Could you check a few things on this model? Use its own coordinates, in mm. Give positions to 0.01 mm unless a question says otherwise; leave off trailing zeros. Use a Markdown table: item, result. Add a question column.
Item 1: If I drill on L1, parallel to X at y = 0.85, z = 8.89; L2, parallel to X at y = 0.15, z = 8.5; L3, parallel to X at y = 0.25, z = -10.5, over which ranges is the centre line in solid material (lowest first)? Write a range as from..to.
Item 2: I'm going to push a flat-ended pin straight in: pin 1 Ø0.8 at (x, z) = (23.37, 2.43) entering from -Y. Where does the tip first touch, or does it pass through?
Item 3: Suppose I cut it at A-A on y = 0.9. Count the separate pieces of the cut face and the enclosed holes in it, plus the area to 3 significant figures.
Item 4: If we mould it in two halves opening along Z, with no side actions, what happens to faces 1 (the face through (-20.32, 0.77, -2.68)), 2 (the face through (0, 1, 11.43)), 3 (the face through (25.4, 1, 0))? For each: released by +Z, released by -Z, zero draft, split by the parting line, or undercut.
from build123d import *

# Parameters (mm, degrees)
SKETCH1_W                 = 50.8
SKETCH1_H                 = 22.86
BOSS_EXTRUDE1_DEPTH       = 1.57
F_1_16_0_1_DOWEL_HOLE1_D  = 2.54
FILLET1_R                 = 2.54
F_1_16_0_04_DOWEL_HOLE3_D = 1.016
LPATTERN6_COUNT           = 4
LPATTERN6_PITCH           = 2.54
LPATTERN6_COUNT_DIR2      = 2
LPATTERN6_PITCH_DIR2      = 2.54
LPATTERN7_COUNT           = 2
LPATTERN7_PITCH           = 2.54
LPATTERN7_COUNT_DIR2      = 4
LPATTERN7_PITCH_DIR2      = 2.54
LPATTERN8_COUNT           = 2
LPATTERN8_PITCH           = 41.656
LPATTERN8_COPY_1_D        = 1.016
LPATTERN8_COPY_2_D        = 1.016
LPATTERN8_COPY_3_D        = 1.016
LPATTERN8_COPY_4_D        = 1.016
LPATTERN8_COPY_5_D        = 1.016
LPATTERN8_COPY_6_D        = 1.016
LPATTERN8_COPY_7_D        = 1.016
LPATTERN8_COPY_8_D        = 1.016
LPATTERN8_COPY_9_D        = 1.016
LPATTERN8_COPY_10_D       = 1.016
LPATTERN8_COPY_11_D       = 1.016
LPATTERN8_COPY_12_D       = 1.016
LPATTERN8_COPY_13_D       = 1.016
LPATTERN8_COPY_14_D       = 1.016


with BuildPart() as part:
    # Sketch1 → Boss-Extrude1 (new body)
    with BuildSketch(Plane(origin=(0, 0, 0), x_dir=(1, 0, 0), z_dir=(0, 1, 0))):
        Rectangle(SKETCH1_W, SKETCH1_H)
    extrude(amount=BOSS_EXTRUDE1_DEPTH)

    # 1/16 (0.1) Dowel Hole1 (through all)
    with Locations(Plane(origin=(0, 1.57, 0), x_dir=(1, 0, 0), z_dir=(0, 1, 0))):
        with Locations((-22.86, 8.89), (22.86, 8.89), (22.86, -8.89), (-22.86, -8.89)):
            Hole(F_1_16_0_1_DOWEL_HOLE1_D / 2)

    # Fillet1
    fillet1_edges = [part.edges().sort_by_distance(p)[0] for p in [
        (25.4, 0.785, 11.43),
        (-25.4, 0.785, 11.43),
        (-25.4, 0.785, -11.43),
        (25.4, 0.785, -11.43),
    ]]
    fillet(fillet1_edges, radius=FILLET1_R)

    # 1/16 (0.04) Dowel Hole3 (through all)
    with Locations(Plane(origin=(0, 1.57, 0), x_dir=(1, 0, 0), z_dir=(0, 1, 0))):
        with Locations((-20.828, -4.965370827)):
            f_1_16_0_04_dowel_hole3 = Hole(F_1_16_0_04_DOWEL_HOLE3_D / 2)

    # LPattern6: 1_16 _0.04_ Dowel Hole3 4 × 2
    with Locations(*[(-j * LPATTERN6_PITCH_DIR2, 0, -i * LPATTERN6_PITCH) for i in range(LPATTERN6_COUNT) for j in range(LPATTERN6_COUNT_DIR2) if (i, j) != (0, 0)]):
        add(f_1_16_0_04_dowel_hole3, mode=Mode.SUBTRACT)

    # LPattern7: 1_16 _0.04_ Dowel Hole3 2 × 4
    with Locations(*[(i * LPATTERN7_PITCH, 0, -j * LPATTERN7_PITCH_DIR2) for i in range(LPATTERN7_COUNT) for j in range(LPATTERN7_COUNT_DIR2) if (i, j) != (0, 0)]):
        add(f_1_16_0_04_dowel_hole3, mode=Mode.SUBTRACT)

    # LPattern8: 1/16 (0.04) Dowel Hole3 ×2
    with Locations(*[(i * LPATTERN8_PITCH, 0, 0) for i in range(1, LPATTERN8_COUNT)]):
        add(f_1_16_0_04_dowel_hole3, mode=Mode.SUBTRACT)

    # LPattern8 copy 1 (through all)
    with Locations(Plane(origin=(39.116, 1.57, 0), x_dir=(1, 0, 0), z_dir=(0, 1, 0))):
        with Locations((-20.828, -4.965370827)):
            Hole(LPATTERN8_COPY_1_D / 2)

    # LPattern8 copy 2 (through all)
    with Locations(Plane(origin=(41.656, 1.57, -2.54), x_dir=(1, 0, 0), z_dir=(0, 1, 0))):
        with Locations((-20.828, -4.965370827)):
            Hole(LPATTERN8_COPY_2_D / 2)

    # LPattern8 copy 3 (through all)
    with Locations(Plane(origin=(39.116, 1.57, -2.54), x_dir=(1, 0, 0), z_dir=(0, 1, 0))):
        with Locations((-20.828, -4.965370827)):
            Hole(LPATTERN8_COPY_3_D / 2)

    # LPattern8 copy 4 (through all)
    with Locations(Plane(origin=(41.656, 1.57, -5.08), x_dir=(1, 0, 0), z_dir=(0, 1, 0))):
        with Locations((-20.828, -4.965370827)):
            Hole(LPATTERN8_COPY_4_D / 2)

    # LPattern8 copy 5 (through all)
    with Locations(Plane(origin=(39.116, 1.57, -5.08), x_dir=(1, 0, 0), z_dir=(0, 1, 0))):
        with Locations((-20.828, -4.965370827)):
            Hole(LPATTERN8_COPY_5_D / 2)

    # LPattern8 copy 6 (through all)
    with Locations(Plane(origin=(41.656, 1.57, -7.62), x_dir=(1, 0, 0), z_dir=(0, 1, 0))):
        with Locations((-20.828, -4.965370827)):
            Hole(LPATTERN8_COPY_6_D / 2)

    # LPattern8 copy 7 (through all)
    with Locations(Plane(origin=(39.116, 1.57, -7.62), x_dir=(1, 0, 0), z_dir=(0, 1, 0))):
        with Locations((-20.828, -4.965370827)):
            Hole(LPATTERN8_COPY_7_D / 2)

    # LPattern8 copy 8 (through all)
    with Locations(Plane(origin=(41.656, 1.57, -2.54), x_dir=(1, 0, 0), z_dir=(0, 1, 0))):
        with Locations((-20.828, -4.965370827)):
            Hole(LPATTERN8_COPY_8_D / 2)

    # LPattern8 copy 9 (through all)
    with Locations(Plane(origin=(41.656, 1.57, -5.08), x_dir=(1, 0, 0), z_dir=(0, 1, 0))):
        with Locations((-20.828, -4.965370827)):
            Hole(LPATTERN8_COPY_9_D / 2)

    # LPattern8 copy 10 (through all)
    with Locations(Plane(origin=(41.656, 1.57, -7.62), x_dir=(1, 0, 0), z_dir=(0, 1, 0))):
        with Locations((-20.828, -4.965370827)):
            Hole(LPATTERN8_COPY_10_D / 2)

    # LPattern8 copy 11 (through all)
    with Locations(Plane(origin=(44.196, 1.57, 0), x_dir=(1, 0, 0), z_dir=(0, 1, 0))):
        with Locations((-20.828, -4.965370827)):
            Hole(LPATTERN8_COPY_11_D / 2)

    # LPattern8 copy 12 (through all)
    with Locations(Plane(origin=(44.196, 1.57, -2.54), x_dir=(1, 0, 0), z_dir=(0, 1, 0))):
        with Locations((-20.828, -4.965370827)):
            Hole(LPATTERN8_COPY_12_D / 2)

    # LPattern8 copy 13 (through all)
    with Locations(Plane(origin=(44.196, 1.57, -5.08), x_dir=(1, 0, 0), z_dir=(0, 1, 0))):
        with Locations((-20.828, -4.965370827)):
            Hole(LPATTERN8_COPY_13_D / 2)

    # LPattern8 copy 14 (through all)
    with Locations(Plane(origin=(44.196, 1.57, -7.62), x_dir=(1, 0, 0), z_dir=(0, 1, 0))):
        with Locations((-20.828, -4.965370827)):
            Hole(LPATTERN8_COPY_14_D / 2)


solid = part.part
Findings below:
| question | item | result |
|---|---|---|
| 1 | L1 | x = -25.4..-24.13, -21.59..21.59, 24.13..25.4 |
| 1 | L2 | x = -25.4..-24.07, -21.65..21.65, 24.07..25.4 |
| 1 | L3 | x = -24.82..24.82 |
| 2 | pin 1 | passes through |
| 3 | separate pieces | 1 |
| 3 | enclosed holes | 28 |
| 3 | area | 1,120 mm^2 |
| 4 | face 1 | undercut |
| 4 | face 2 | released by +Z |
| 4 | face 3 | zero draft |
